Build history of the part. All positions in model axes, mm. Face numbers are marked on the shaded views. A direction names the side the tool comes from. Coordinates: 2 decimals unless noted, no trailing zeros. Loops run counter-clockwise (first coordinate to the right, second up) from the corner with the lowest first, then second, coordinate; pieces in that order, holes last. Notation, with made-up numbers: (-25, 77.5) - (16, 77.5) arc R21 cw to (16, 109.5) - close; hole circle Ø1 at (27.5, -5.75). An arc over 180 degrees is marked (long way). One line per item, written item: value.
```python
from build123d import *

# Parameters (mm, degrees)
LANGUETTE_R        = 0.598025677
LANGUETTE_R_2      = 0.602747005
BOSS_EXTRU_1_DEPTH = 0.25
CONTACTS_W         = 8.310994675
CONTACTS_H         = 2.119060631
BOSS_EXTRU_2_DEPTH = 0.26
BOSS_EXTRU_3_DEPTH = 1.5
ESQUISSE7_R        = 17.010621832
BOSS_EXTRU_4_DEPTH = 0.25


with BuildPart() as part:
    # languette → Boss.-Extru.1 (new body)
    with BuildSketch(Plane.XY):
        with BuildLine():
            Line((-6.595613447, -8.888713039), (-5.615374712, -7.488966567))
            Line((-5.615374712, -7.488966567), (-5.615374712, -5.383882856))
            ThreePointArc((-5.615374712, -5.383882856), (-5.468928102, -5.030329465), (-5.115374712, -4.883882856))
            Line((-5.115374712, -4.883882856), (5.403372294, -4.883882856))
            ThreePointArc((5.403372294, -4.883882856), (5.756925685, -5.030329465), (5.903372294, -5.383882856))
            Line((5.903372294, -5.383882856), (5.903372294, -15.510913379))
            Line((5.903372294, -15.510913379), (-6.595613447, -15.510913379))
            Line((-6.595613447, -15.510913379), (-6.595613447, -8.888713039))
        make_face()
        with Locations((-5.236276709, -9.190047348)):
            Circle(LANGUETTE_R, mode=Mode.SUBTRACT)
        with Locations((4.736916901, -9.190047348)):
            Circle(LANGUETTE_R_2, mode=Mode.SUBTRACT)
    extrude(amount=-BOSS_EXTRU_1_DEPTH)

    # contacts → Boss.-Extru.2 (add)
    with BuildSketch(Plane.XY):
        with Locations((0.143998792, -5.943413172)):
            Rectangle(CONTACTS_W, CONTACTS_H)
    extrude(amount=-BOSS_EXTRU_2_DEPTH)

    # Esquisse6 → Boss.-Extru.3 (add)
    with BuildSketch(Plane.XY):
        with BuildLine():
            Line((-6.595613447, -15.510913379), (-8.043725423, -11.761859924))
            ThreePointArc((-8.043725423, -11.761859924), (-15.286364086, -4.654195518), (-17.723977577, 5.196324701))
            ThreePointArc((-17.723977577, 5.196324701), (2.671119001, 22.861069139), (17.103268201, 0.063783556))
            ThreePointArc((17.103268201, 0.063783556), (13.761328931, -6.761125674), (8.03938861, -11.761859924))
            Line((8.03938861, -11.761859924), (6.626148003, -15.510913379))
            Line((6.626148003, -15.510913379), (-6.595613447, -15.510913379))
        make_face()
    extrude(amount=BOSS_EXTRU_3_DEPTH)

    # Esquisse7 → Boss.-Extru.4 (add)
    with BuildSketch(Plane.XY.offset(1.5)):
        with Locations((0.07593762, 5.251269776)):
            Circle(ESQUISSE7_R)
    extrude(amount=BOSS_EXTRU_4_DEPTH)


solid = part.part
```
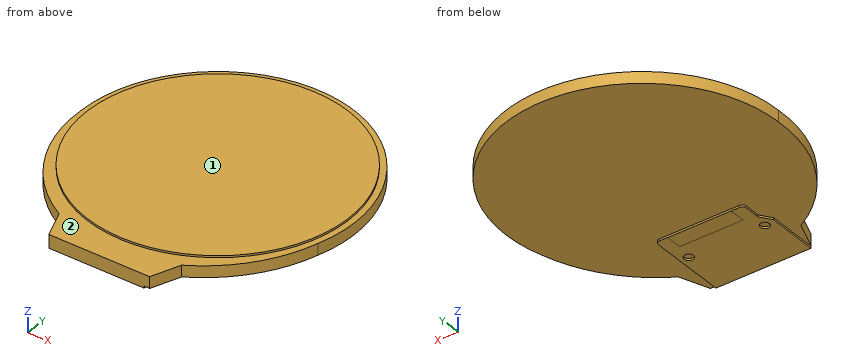
Item 1: Cut at D-D, the plane y = 1. Write the cut outline in (x, z).
Check result:
outline: (-17.39, 0) - (17.36, 0) - (17.36, 1.5) - (16.55, 1.5) - (16.55, 1.75) - (-16.39, 1.75) - (-16.39, 1.5) - (-17.39, 1.5) - close
Item 2: Tool access for the marked faces 1 and 2: list every direction of +Z, -Z, +X, -X, +Y, -Y with a clear straight run to the whole face (end or side of a thin tool).
Check result:
face 1: +Z, +X, -X, +Y, -Y
face 2: +Z
Item 3: Probe probe 1 along Z at (x, y) = (-11, 4.5); probe 2 along Y at (x, z) = (-3, -0.1); probe 3 along Z at (x, y) = (13, 17). List the from-to ranges inside material, lowest first. Write a range as from..to.
Check result:
probe 1: z = 0..1.75
probe 2: y = -15.51..-4.88
probe 3: z = 0..1.5
Item 4: Cut at B-B, the plane y = 16.5. Write the cut outline in (x, z).
Check result:
outline: (-13.72, 0) - (13.87, 0) - (13.87, 1.5) - (12.84, 1.5) - (12.84, 1.75) - (-12.68, 1.75) - (-12.68, 1.5) - (-13.72, 1.5) - close
Item 5: Drop flat-ended pins along their axis: P1, Ø0.7, axis at x = 4.74, y = -9.19, coming from the -Z side; P2, Ø5.5, axis at x = 0, y = -13, coming from the -Z side. Give the stop position or say it passes through.
Check result:
P1: stops at z = 0
P2: stops at z = -0.25
Item 6: Cut at C-C, the plane z = 0.85. Write the cut outline in (x, y).
Check result:
outline: (-17.72, 5.2) arc R18.61 ccw to (-8.04, -11.76) - (-6.6, -15.51) - (6.63, -15.51) - (8.04, -11.76) arc R19.26 ccw to (17.1, 0.06) arc R17.8 ccw (long way) to start
